Input: part model. Units: mm. Frame: model coordinates. Coordinates: 2 decimals unless noted, no trailing zeros. Order: outer loops, then holes, each group sorted by start corner. A loop starts at its lowest first (then second) coordinate and runs counter-clockwise, first axis right, second up. Notation, with made-up numbers: (-2, 31) - (9, 31) arc R11 ccw to (9, 45) - close; hole circle Ø10 at (-12.75, 58). An arc over 180 degrees is marked (long way). Answer as CSV lines item,"result". Start each with the question number.
Item 1: Section A-A (y = 66). Output: boundary loops of the cut face in (x, z), and give its area (3 significant figures).
Item 2: Section B-B (x = 33.5). Output: boundary loops of the cut face in (y, z), and give its area (3 significant figures).
Item 3: First-contact query: pin 1 (3 mm diameter, centred on y = -3, z = 3.5, fed in from +X); pin 2 (3 mm diameter, centred on y = -4, z = 3.5, fed in from -X); pin 3 (1.8 mm diameter, centred on y = 32.5, z = 3.5, fed in from +X). Flat tips, straight axial feed; report the tip coordinate or a pass-through.
Item 4: Material intervals for line 1 along X through (y, z) = (-1, 1.2); line 2 along Y through (x, z) = (113.5, 3.65); line 3 along X through (y, z) = (28, 2.5), sorted ascending.
Autodesk Inventor part; units mm, degrees
ref_plane "YZ Plane" through (0, 0, 0) normal (1, 0, 0) x (0, 1, 0)
ref_plane "XZ Plane" through (0, 0, 0) normal (0, 1, 0) x (-1, 0, 0)
ref_plane "XY Plane" through (0, 0, 0) normal (0, 0, 1) x (1, 0, 0)
ref_plane "Work Plane1" through (0, 0, 0) normal (0, 0, 1) x (1, 0, 0)
sketch "Sketch1" plane through (0, 0, 0) normal (0, 0, 1) x (1, 0, 0)
  line L0 (0, 0) -> (30, 0)
  line L1 (0, 0) -> (0, -6)
  line L2 (30, -6) -> (0, -6)
  line L3 (30, 0) -> (30, -6)
  line L4 (60, 0) -> (90, 0)
  line L5 (60, 0) -> (60, -6)
  line L6 (90, -6) -> (60, -6)
  line L7 (90, 0) -> (90, -6)
  line L8 (120, 0) -> (150, 0)
  line L9 (120, 0) -> (120, -6)
  line L10 (150, -6) -> (120, -6)
  line L11 (150, 0) -> (150, -6)
  line L12 (180, 0) -> (210, 0)
  line L13 (180, 0) -> (180, -6)
  line L14 (210, -6) -> (180, -6)
  line L15 (210, 0) -> (210, -6)
  line L16 (240, 0) -> (270, 0)
  line L17 (240, 0) -> (240, -6)
  line L18 (270, -6) -> (240, -6)
  line L19 (270, 0) -> (270, -6)
  line L20 (300, 0) -> (330, 0)
  line L21 (300, 0) -> (300, -6)
  line L22 (330, -6) -> (300, -6)
  line L23 (330, 0) -> (330, -6)
  line L24 (330, 0) -> (330, -6)
  line L25 (330, -6) -> (365, -6)
  line L26 (365, -6) -> (365, 0)
  line L27 (365, 0) -> (330, 0)
  line L28 (300, -6) -> (300, 0)
  line L29 (300, 0) -> (270, 0)
  line L30 (270, 0) -> (270, -6)
  line L31 (270, -6) -> (300, -6)
  line L32 (210, 0) -> (210, -6)
  line L33 (210, -6) -> (240, -6)
  line L34 (240, -6) -> (240, 0)
  line L35 (240, 0) -> (210, 0)
  line L36 (150, 0) -> (150, -6)
  line L37 (150, -6) -> (180, -6)
  line L38 (180, -6) -> (180, 0)
  line L39 (180, 0) -> (150, 0)
  line L40 (120, -6) -> (120, 0)
  line L41 (120, 0) -> (90, 0)
  line L42 (90, 0) -> (90, -6)
  line L43 (90, -6) -> (120, -6)
  line L44 (30, 0) -> (30, -6)
  line L45 (30, -6) -> (60, -6)
  line L46 (60, -6) -> (60, 0)
  line L47 (60, 0) -> (30, 0)
  line L48 (0, -6) -> (0, 0)
  line L49 (0, 0) -> (-35, 0)
  line L50 (-35, -6) -> (-35, 0)
  line L51 (-35, -6) -> (0, -6)
  line L52 (0, 0) -> (-35, 0)
  line L53 (30, 0) -> (60, 0)
  line L54 (90, 0) -> (120, 0)
  line L55 (150, 0) -> (180, 0)
  line L56 (210, 0) -> (240, 0)
  line L57 (270, 0) -> (300, 0)
  line L58 (330, 0) -> (365, 0)
  line L59 (330, 0) -> (330, -6)
  line L60 (300, 0) -> (300, -6)
  line L61 (330, -6) -> (300, -6)
  line L62 (270, 0) -> (270, -6)
  line L63 (240, -6) -> (240, 0)
  line L64 (240, -6) -> (270, -6)
  line L65 (210, 0) -> (210, -6)
  line L66 (180, -6) -> (210, -6)
  line L67 (180, -6) -> (180, 0)
  line L68 (150, 0) -> (150, -6)
  line L69 (120, -6) -> (150, -6)
  line L70 (120, -6) -> (120, 0)
  line L71 (90, 0) -> (90, -6)
  line L72 (90, -6) -> (60, -6)
  line L73 (60, 0) -> (60, -6)
  line L74 (30, 0) -> (30, -6)
  line L75 (0, 0) -> (0, -6)
  line L76 (30, -6) -> (0, -6)
  line L77 (-35, 0) -> (-35, 100)
  line L78 (-35, 100) -> (365, 100)
  line L79 (365, 0) -> (365, 100)
  dimension "d0" = 100
extrude "Plate1" add sketch "Sketch1" along normal blind 6 contours L49 L77 L78 L79 L27 L20 L29 L16 L35 L12 L39 L8 L41 L4 L47 L0 | L0 L3 L2 L1 | L4 L7 L6 L5 | L8 L11 L10 L9 | L23 L22 L21 L20 | L12 L15 L14 L13 | L19 L18 L17 L16
sketch "Sketch2" plane through (0, 0, 0) normal (0, 0, -1) x (-1, 0, 0)
  line L0 (-359, 60) -> (-359, 80)
  line L1 (-365, 80) -> (-359, 80)
  line L2 (-365, 80) -> (-365, 60)
  line L3 (-365, 60) -> (-359, 60)
  line L4 (-359, 20) -> (-359, 40)
  line L5 (-365, 40) -> (-359, 40)
  line L6 (-365, 40) -> (-365, 20)
  line L7 (-365, 20) -> (-359, 20)
  line L8 (29, 80) -> (29, 60)
  line L9 (35, 60) -> (29, 60)
  line L10 (35, 60) -> (35, 80)
  line L11 (35, 80) -> (29, 80)
  line L12 (29, 40) -> (29, 20)
  line L13 (35, 20) -> (29, 20)
  line L14 (35, 20) -> (35, 40)
  line L15 (35, 40) -> (29, 40)
  point P0 (0, 0)
extrude "Cut1" cut sketch "Sketch2" against normal blind 6
equation "\"d2\" = Thickness"
equation "\"d1\" = Thickness"
equation "\"BendRadius\" = Thickness"
equation "\"BendReliefWidth\" = Thickness"
equation "\"BendReliefDepth\" = 0.5 * Thickness"
equation "\"CornerReliefSize\" = 4 * Thickness"
equation "\"MinimumRemnant\" = 2 * Thickness"
equation "\"TransitionRadius\" = BendRadius"
equation "\"JacobiRadiusSize\" = BendRadius"
equation "\"GapSize\" = Thickness"
properties part number "zijkant electronica" material "Wood (Birch)"
Determined:
1,outline,"(-29, 0) - (359, 0) - (359, 6) - (-29, 6) - close"
1,area,"2,330 mm^2"
2,outline,"(0, 0) - (100, 0) - (100, 6) - (0, 6) - close"
2,area,"600 mm^2"
3,pin 1,"stops at x = 330"
3,pin 2,"stops at x = 0"
3,pin 3,"stops at x = 359"
4,line 1,"x = 0 to 30, 60 to 90, 120 to 150, 180 to 210, 240 to 270, 300 to 330"
4,line 2,"y = 0 to 100"
4,line 3,"x = -29 to 359"
